The listing builds one solid part. Answer for the finished solid, in the listing's coordinates (mm). A direction names the side the tool comes from. Coordinates: 2 decimals unless noted, no trailing zeros. Order: outer loops, then holes, each group sorted by start corner. A loop starts at its lowest first (then second) coordinate and runs counter-clockwise, first axis right, second up.
from build123d import *

# Parameters (mm, degrees)
F1_DEPTH = 18
F2_R     = 4
F3_DEPTH = 1.4


with BuildPart() as f1:
    # F0 (on Top) → F1 (new body)
    with BuildSketch(Plane.XY):
        with BuildLine():
            ThreePointArc((0, 10), (10, 0), (0, -10))
            Line((0, -10), (-17.59439, -7.979329))
            ThreePointArc((-17.59439, -7.979329), (-16.838188, -8.866441), (-16.566426, -10))
            ThreePointArc((-16.566426, -10), (-17.237867, -11.704809), (-18.891523, -12.493874))
            Line((-18.891523, -12.493874), (-0.004054, -12.499999))
            ThreePointArc((-0.004054, -12.499999), (12.5, 0), (-0.004054, 12.499999))
            Line((-0.004054, 12.499999), (-19.066426, 12.5))
            ThreePointArc((-19.066426, 12.5), (-17.298659, 11.767767), (-16.566426, 10))
            ThreePointArc((-16.566426, 10), (-16.838188, 8.866441), (-17.59439, 7.979329))
            Line((-17.59439, 7.979329), (0, 10))
        make_face()
        with BuildLine():
            ThreePointArc((-16.566426, -10), (-16.838188, -8.866441), (-17.59439, -7.979329))
            ThreePointArc((-17.59439, -7.979329), (-21.469212, -9.309624), (-18.891523, -12.493874))
            ThreePointArc((-18.891523, -12.493874), (-17.237867, -11.704809), (-16.566426, -10))
        make_face()
        with BuildLine():
            ThreePointArc((-19.066426, 12.5), (-21.443575, 9.225945), (-17.59439, 7.979329))
            ThreePointArc((-17.59439, 7.979329), (-16.838188, 8.866441), (-16.566426, 10))
            ThreePointArc((-16.566426, 10), (-17.298659, 11.767767), (-19.066426, 12.5))
        make_face()
    extrude(amount=F1_DEPTH)

    # F2 (on face) → F3 (cut)
    with BuildSketch(Plane(origin=(-0.004054, -12.499999, 0), x_dir=(1, -0.000324, 0), z_dir=(-0.000324, -1, 0))):
        with Locations((-13.686376, 4.757359)):
            Circle(F2_R)
        with Locations((-13.686376, 13.242641)):
            Circle(F2_R)
        with Locations((-5.201095, 13.242641)):
            Circle(F2_R)
        with Locations((-5.201095, 4.757359)):
            Circle(F2_R)
    extrude(amount=-F3_DEPTH, mode=Mode.SUBTRACT)


solid = f1.part
(1) Find section A-A on x = 6. Determine the outline of the cut face in (y, z).
(2) A tool of negligible diameter and unlimited length cuts with its end or side. For faces 1 (the flat face through (-9, 12.5, 9)), 2 (the cylindrical face through (10, 0, 9)), from which of +Z, -Z, +X, -X, +Y, -Y can it reach the whole face along a straight path? Write none if from no direction.
(3) Given pin 1 Ø10.5 at (x, z) = (-13.69, 4.76) entering from -Y; pin 2 Ø6 at (y, z) = (-8.5, 2.5) entering from +X (3 decimals); pin 3 Ø3 at (x, z) = (5.5, 15) entering from +Y, each flat-ended and moving along its own axis, determine where each tip first touches the part or whether it passes through.
(4) Find section C-C on y = 0. Determine the outline of the cut face in (x, z).
(5) Find the intervals of material crossed by probe 1 along Y at (x, z) = (-10, 14); probe 2 along Y at (x, z) = (-19, 3); probe 3 along X at (y, z) = (-1.5, 10.25), in increasing order.
(6) Find section D-D on z = 13.75. Determine the outline of the cut face in (x, y), then the cut area to 3 significant figures.
(7) The mould has two halves that part along Z. Classify faces 3 (the flat face through (-8.92, 8.976, 8.874)), 4 (the flat face through (-8.4, -9.2, 18)), 5 (the cylindrical face through (-9.875, -11.807, 5.959)), 6 (the cylindrical face through (-6.07, -11.81, 0.85)): pulls with the +Z half, pulls with the -Z half, needs draft (parallel to the pull), parting line crosses it, or undercut.
(8) Find section B-B on z = 10.5. Determine the outline of the cut face in (x, y), then the cut area to 3 significant figures.
Resolved:
1. outline: (-10.97, 0) - (-8, 0) - (-8, 18) - (-10.97, 18) - close; (8, 0) - (10.97, 0) - (10.97, 18) - (8, 18) - close
2. face 1: +Z, -Z, +X, -X, +Y
2. face 2: +Z, -Z
3. pin 1: stops at y = -12.5
3. pin 2: stops at x = 11.225
3. pin 3: stops at y = 11.84
4. outline: (10, 0) - (12.5, 0) - (12.5, 18) - (10, 18) - close
5. probe 1: y = -11.1 to -8.85, 8.85 to 12.5
5. probe 2: y = -12.5 to -7.5, 7.5 to 12.5
5. probe 3: x = 9.89 to 12.41
6. outline: (-19.07, 12.5) arc R2.5 ccw (long way) to (-17.59, 7.98) - (0, 10) arc R10 cw to (0, -10) - (-17.59, -7.98) arc R2.5 ccw (long way) to (-18.89, -12.49) - (-17.66, -12.49) - (-17.66, -11.09) - (-9.72, -11.1) - (-9.72, -12.5) - (-9.17, -12.5) - (-9.17, -11.1) - (-1.24, -11.1) - (-1.24, -12.5) - (0, -12.5) arc R12.5 ccw to (0, 12.5) - close
6. area: 224 mm2
7. face 3: needs draft
7. face 4: pulls with the +Z half
7. face 5: undercut
7. face 6: undercut
8. outline: (-19.07, 12.5) arc R2.5 ccw (long way) to (-17.59, 7.98) - (0, 10) arc R10 cw to (0, -10) - (-17.59, -7.98) arc R2.5 ccw (long way) to (-18.89, -12.49) - (-16.6, -12.49) - (-16.6, -11.09) - (-10.78, -11.1) - (-10.78, -12.5) - (-8.12, -12.5) - (-8.12, -11.1) - (-2.29, -11.1) - (-2.29, -12.5) - (0, -12.5) arc R12.5 ccw to (0, 12.5) - close
8. area: 229 mm2
